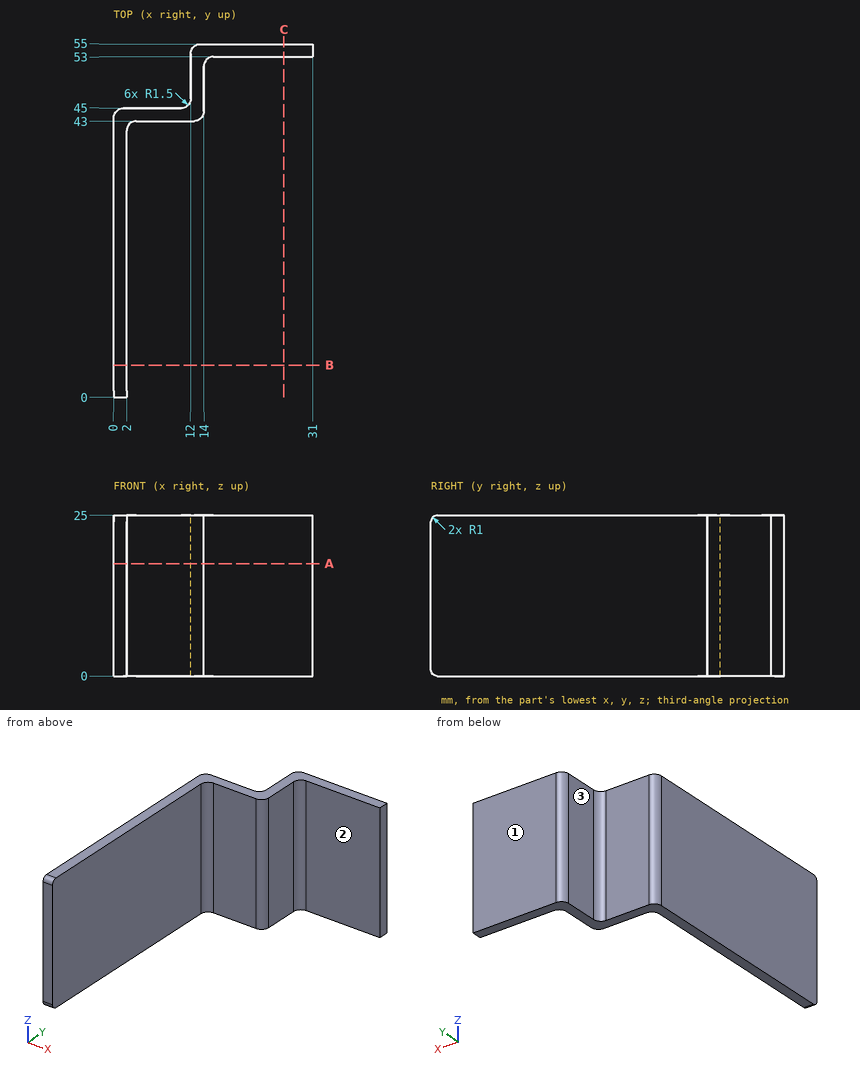
Design review of the part shown in the three views and the two pictorial views. Dimensions are in mm from the part's minimum x, y and z. A direction names the side the tool comes from. Round coordinates to 2 decimals unless told otherwise and drop trailing zeros. Write each loop counter-clockwise with the first axis right and the second up, starting at its lowest first coordinate (ties: lowest second). Pieces come first, ordered by that corner, then holes. Notation, with made-up numbers: (78, 74) -> (100, 74) arc R29 ccw to (100, 94) -> close; hole circle Ø4 at (-28, 84). An arc over 180 degrees is marked (long way). Answer as a JSON object with one key per item and string values.
1. Clearance check with flat-ended pins moving along their axes: pin 1 (4.5 mm diameter, centred on x = 22, z = 18.5, fed in from -Y); pin 2 (7.5 mm diameter, centred on y = 50, z = 11.5, fed in from -X); pin 3 (6 mm diameter, centred on x = 9.5, z = 11.5, fed in from -Y). State where each tip first meets the part, or that it passes through.
Results found:
{"pin 1": "stops at y = 53", "pin 2": "stops at x = 11.98", "pin 3": "stops at y = 43"}
2. To check wall thickness, follow line 1 along X through (y, z) = (13, 19.5); line 2 along Y through (x, z) = (24.5, 20); line 3 along Y through (x, z) = (4.5, 8.75). State the ranges of each line that lie inside material, in increasing order.
Results found:
{"line 1": "x = 0 to 2", "line 2": "y = 53 to 55", "line 3": "y = 43 to 45"}
3. Machinability: for the marked faces 1, 2 and 3, which of the approach directions +Z, -Z, +X, -X, +Y, -Y give a long, thin tool a straight path to every point of the face, cutting with its end or side? Answer none if there is none.
Results found:
{"face 1": "+Z, -Z, +X, -X, +Y", "face 2": "+Z, -Z, +X, -Y", "face 3": "+Z, -Z, -X, +Y"}
4. We need section B-B on y = 5. State the section outline as (x, z) points.
Results found:
{"outline": "(0, 0) -> (2, 0) -> (2, 25) -> (0, 25) -> close"}
5. We need section C-C on x = 26.5. State the section outline as (y, z) points.
Results found:
{"outline": "(53, 0) -> (55, 0) -> (55, 25) -> (53, 25) -> close"}
6. We need section A-A on z = 17.5. State the section outline as (x, y) points, and give its area (3 significant figures).
Results found:
{"outline": "(0, 0) -> (2, 0) -> (2, 41.5) arc R1.5 cw to (3.5, 43) -> (12.5, 43) arc R1.5 ccw to (14, 44.5) -> (14, 51.5) arc R1.5 cw to (15.5, 53) -> (31, 53) -> (31, 55) -> (13.5, 55) arc R1.5 ccw to (12, 53.5) -> (12, 46.5) arc R1.5 cw to (10.5, 45) -> (1.5, 45) arc R1.5 ccw to (0, 43.5) -> close", "area": "168 mm^2"}
